For this review, take the finished solid that the model builds, in its own axes (mm). Face numbers are marked on the shaded views. A direction names the side the tool comes from. Coordinates: 2 decimals unless noted, no trailing zeros. Order: outer loops, then holes, each group sorted by start corner. A loop starts at its lowest first (then second) coordinate and runs counter-clockwise, first axis right, second up. Notation, with made-up numbers: M 9.25,12.25 L 56.25,12.25 A15 cw 56.25,27.25 Z; hole C 60,88 d11. An arc over 180 degrees is marked long. Use one line per item in the form item = value. Start each with the question number.
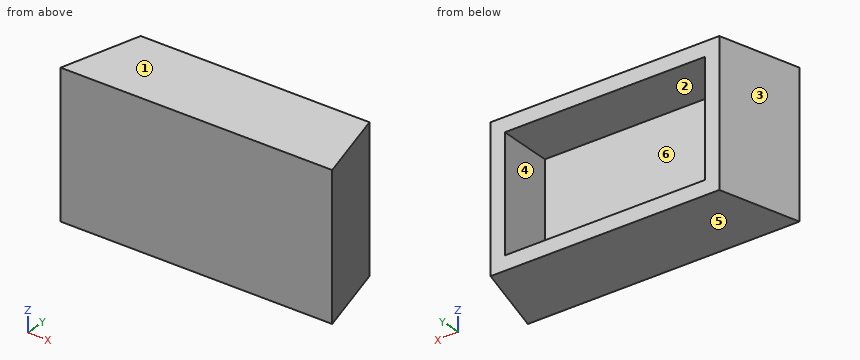
```python
from build123d import *

# Parameters (mm, degrees)
SKETCH003_W      = 14
SKETCH003_H      = 8
EXTRUDE002_DEPTH = 3.75
EXTRUDE001_DEPTH = 10


with BuildPart() as extrude002:
    # Sketch003 (on Face2 of Extrude001) → Extrude002 (new body, symmetric)
    with BuildSketch(Plane(origin=(0, 7.5, 0), x_dir=(-1, 0, 0), z_dir=(0, 1, 0))):
        with Locations((0, 5)):
            Rectangle(SKETCH003_W, SKETCH003_H)
    extrude(amount=EXTRUDE002_DEPTH, both=True)


with BuildPart() as cut:
    # Sketch001 → Extrude001 (new body)
    with BuildSketch(Plane.XY):
        Polygon((-9.5, 2), (-8, 7.5), (8, 7.5), (9.5, 2), align=None)
    extrude(amount=EXTRUDE001_DEPTH)

    # Cut: cut Extrude002
    add(extrude002.part, mode=Mode.SUBTRACT)


solid = cut.part
```
1. Consider section D-D, the plane y = 5.3. Write out the cut boundary in (x, z), plus the area to 3 significant figures.
2. Consider section C-C, the plane x = -5. Write out the cut boundary in (y, z), plus the area to 3 significant figures.
3. The part is to be moulded in two halves that separate along X. For the marked faces 1, 2, 3 and 4, say which applies: pulls with the +X half, pulls with the -X half, needs draft (parallel to the pull), parting line crosses it, or undercut.
4. For pin 1 Ø1.5 at (x, z) = (1, 5) entering from +Y; pin 2 Ø5 at (x, z) = (4.5, 1.5) entering from +Y; pin 3 Ø1.9 at (y, z) = (6.5, 6.5) entering from +X; pin 4 Ø1.5 at (y, z) = (4, 8) entering from +X, all flat-tipped, find the tip position at first contact; note any pin that passes through.
5. Consider section A-A, the plane y = 4.45. Write out the cut boundary in (x, z), plus the area to 3 significant figures.
6. To check wall thickness, follow line 1 (Z direction, x = 3, y = 6.65); line 2 (Y direction, x = -6.75, z = 2.5); line 3 (X direction, y = 5.2, z = 7.75). State the ranges of each line that lie inside material, in increasing order.
7. Tool access review of the marked faces 5 and 6: name each direction out of +Z, -Z, +X, -X, +Y, -Y from which nothing blocks a thin tool from reaching the whole face with its end or side.
8. Consider section B-B, the plane z = 7.5. Write out the cut boundary in (x, y).
Answers follow:
q1.outline = M -8.6,0 L 8.6,0 L 8.6,10 L -8.6,10 Z; hole M -7,1 L 7,1 L 7,9 L -7,9 Z
q1.area = 60.0 mm²
q2.outline = M 2,0 L 7.5,0 L 7.5,1 L 3.75,1 L 3.75,9 L 7.5,9 L 7.5,10 L 2,10 Z
q2.area = 25.0 mm²
q3.face_1 = needs draft
q3.face_2 = undercut
q3.face_3 = pulls with the -X half
q3.face_4 = undercut
q4.pin_1 = 3.75
q4.pin_2 = 7.5
q4.pin_3 = 8.53
q4.pin_4 = 9.16
q5.outline = M -8.83,0 L 8.83,0 L 8.83,10 L -8.83,10 Z; hole M -7,1 L 7,1 L 7,9 L -7,9 Z
q5.area = 64.6 mm²
q6.line_1 = 0 to 1, 9 to 10
q6.line_2 = 2 to 3.75
q6.line_3 = -8.63 to -7, 7 to 8.63
q7.face_5 = -Z, +X, -X, +Y, -Y
q7.face_6 = +Y
q8.outline = M -9.5,2 L 9.5,2 L 8,7.5 L 7,7.5 L 7,3.75 L -7,3.75 L -7,7.5 L -8,7.5 Z
